Can you work these out from the drawing? Everything is in mm from the part's minimum corner. Give positions to 0.01 mm unless a question says otherwise; leave off trailing zeros. Order: outer loops, then holes, each group sorted by start corner. A loop starts at its lowest first (then second) coordinate and runs counter-clockwise, first axis right, second up. Notation, with made-up numbers: (64.25, 6.25) - (74.25, 6.25) arc R27 cw to (74.25, 41.25) - close; hole circle Ø2 at (57.25, 17). An arc over 180 degrees is marked (long way). Answer as a JSON object with one key per item and string values.
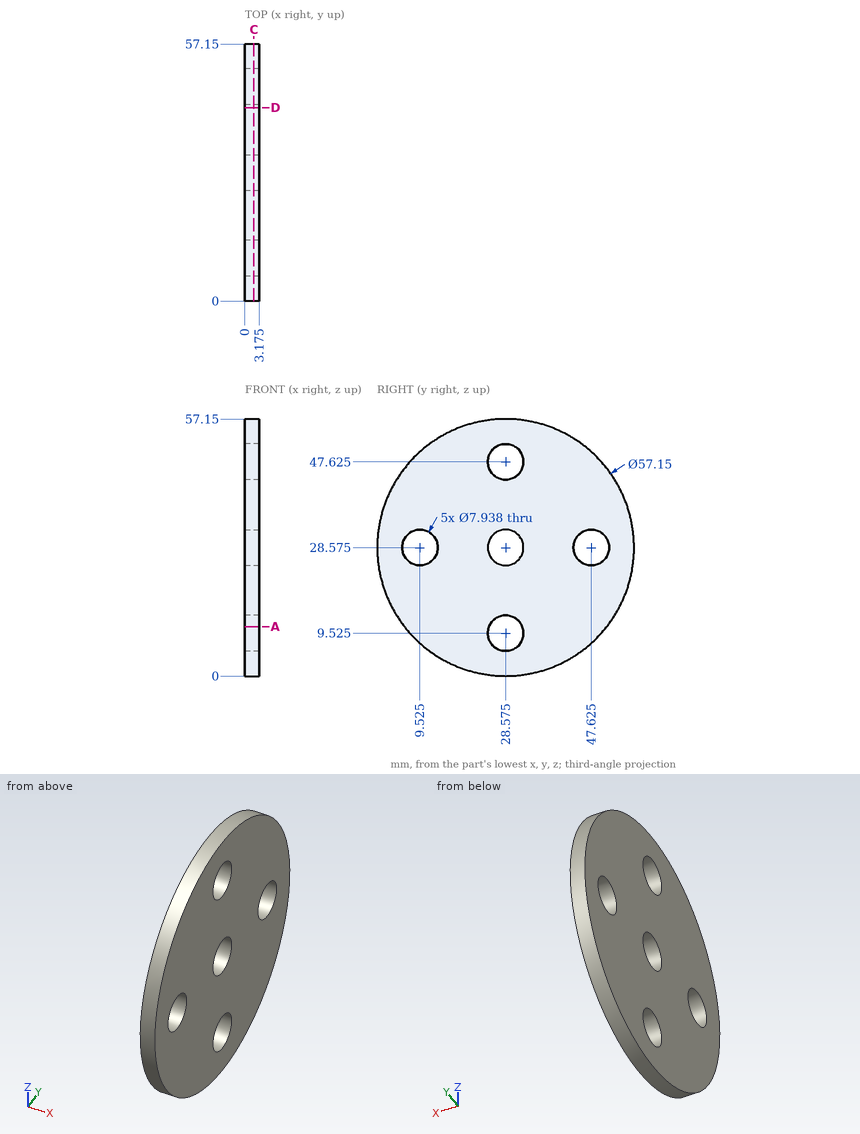
Q1. If we section it at D-D, the plane y = 43: Please give me the cut outline in (x, z) (1 decimal), then the cut area to 3 significant figures.
Recorded:
{"outline": "(0, 3.9) - (3.2, 3.9) - (3.2, 53.2) - (0, 53.2) - close", "area": "157 mm^2"}
Q2. If we section it at C-C, the plane x = 2: Count the separate pieces of the cut face and the enclosed holes in it, then the cut area to 3 significant figures.
Recorded:
{"separate pieces": "1", "enclosed holes": "5", "area": "2,320 mm^2"}
Q3. If we section it at A-A, the plane z = 11: Please give me the cut outline in (x, y) (1 decimal), then the cut area to 3 significant figures.
Recorded:
{"outline": "(0, 6) - (3.2, 6) - (3.2, 24.9) - (0, 24.9) - close; (0, 32.3) - (3.2, 32.3) - (3.2, 51.1) - (0, 51.1) - close", "area": "120 mm^2"}
Q4. I need wall thicknesses on L1, parallel to Z at x = 1.9, y = 50.5; L2, parallel to Z at x = 0.15, y = 21.5; L3, parallel to Y at x = 0.35, z = 46 (1 decimal). Which ranges of each line are inside material? Lowest first, please.
Recorded:
{"L1": "z = 10.25 to 25.84, 31.31 to 46.9", "L2": "z = 0.89 to 56.26", "L3": "y = 5.9 to 25, 32.2 to 51.2"}
